```python
from build123d import *

# Parameters (mm, degrees)
SKETCH_1_R      = 3.4
EXTRUDE_1_DEPTH = 120


with BuildPart() as part:
    # 草图1 → 凸台-拉伸1 (new body)
    with BuildSketch(Plane.XY):
        with BuildLine():
            Line((104, 5.1), (105, 5.1))
            Line((105, 5.1), (105, 12.5))
            ThreePointArc((105, 12.5), (104.267766953, 14.267766953), (102.5, 15))
            Line((102.5, 15), (95.1, 15))
            Line((95.1, 15), (95.1, 14))
            Line((95.1, 14), (94.1, 14))
            Line((94.1, 14), (94.1, 12.6))
            Line((94.1, 12.6), (98.25, 12.6))
            Line((98.25, 12.6), (98.25, 10.014213562))
            Line((98.25, 10.014213562), (94.035786438, 5.8))
            Line((94.035786438, 5.8), (85.964213562, 5.8))
            Line((85.964213562, 5.8), (81.75, 10.014213562))
            Line((81.75, 10.014213562), (81.75, 12.6))
            Line((81.75, 12.6), (85.9, 12.6))
            Line((85.9, 12.6), (85.9, 14))
            Line((85.9, 14), (84.9, 14))
            Line((84.9, 14), (84.9, 15))
            Line((84.9, 15), (65.1, 15))
            Line((65.1, 15), (65.1, 14))
            Line((65.1, 14), (64.1, 14))
            Line((64.1, 14), (64.1, 12.6))
            Line((64.1, 12.6), (68.25, 12.6))
            Line((68.25, 12.6), (68.25, 10.014213562))
            Line((68.25, 10.014213562), (64.035786438, 5.8))
            Line((64.035786438, 5.8), (55.964213562, 5.8))
            Line((55.964213562, 5.8), (51.75, 10.014213562))
            Line((51.75, 10.014213562), (51.75, 12.6))
            Line((51.75, 12.6), (55.9, 12.6))
            Line((55.9, 12.6), (55.9, 14))
            Line((55.9, 14), (54.9, 14))
            Line((54.9, 14), (54.9, 15))
            Line((54.9, 15), (35.1, 15))
            Line((35.1, 15), (35.1, 14))
            Line((35.1, 14), (34.1, 14))
            Line((34.1, 14), (34.1, 12.6))
            Line((34.1, 12.6), (38.25, 12.6))
            Line((38.25, 12.6), (38.25, 10.014213562))
            Line((38.25, 10.014213562), (34.035786438, 5.8))
            Line((34.035786438, 5.8), (25.964213562, 5.8))
            Line((25.964213562, 5.8), (21.75, 10.014213562))
            Line((21.75, 10.014213562), (21.75, 12.6))
            Line((21.75, 12.6), (25.9, 12.6))
            Line((25.9, 12.6), (25.9, 14))
            Line((25.9, 14), (24.9, 14))
            Line((24.9, 14), (24.9, 15))
            Line((24.9, 15), (5.1, 15))
            Line((5.1, 15), (5.1, 14))
            Line((5.1, 14), (4.1, 14))
            Line((4.1, 14), (4.1, 12.6))
            Line((4.1, 12.6), (8.25, 12.6))
            Line((8.25, 12.6), (8.25, 10.014213562))
            Line((8.25, 10.014213562), (4.035786438, 5.8))
            Line((4.035786438, 5.8), (-4.035786438, 5.8))
            Line((-4.035786438, 5.8), (-8.25, 10.014213562))
            Line((-8.25, 10.014213562), (-8.25, 12.6))
            Line((-8.25, 12.6), (-4.1, 12.6))
            Line((-4.1, 12.6), (-4.1, 14))
            Line((-4.1, 14), (-5.1, 14))
            Line((-5.1, 14), (-5.1, 15))
            Line((-5.1, 15), (-12.5, 15))
            ThreePointArc((-12.5, 15), (-14.267766953, 14.267766953), (-15, 12.5))
            Line((-15, 12.5), (-15, 5.1))
            Line((-15, 5.1), (-14, 5.1))
            Line((-14, 5.1), (-14, 4.1))
            Line((-14, 4.1), (-12.6, 4.1))
            Line((-12.6, 4.1), (-12.6, 8.25))
            Line((-12.6, 8.25), (-10.014213562, 8.25))
            Line((-10.014213562, 8.25), (-5.8, 4.035786438))
            Line((-5.8, 4.035786438), (-5.8, -4.035786438))
            Line((-5.8, -4.035786438), (-10.014213562, -8.25))
            Line((-10.014213562, -8.25), (-12.6, -8.25))
            Line((-12.6, -8.25), (-12.6, -4.1))
            Line((-12.6, -4.1), (-14, -4.1))
            Line((-14, -4.1), (-14, -5.1))
            Line((-14, -5.1), (-15, -5.1))
            Line((-15, -5.1), (-15, -12.5))
            ThreePointArc((-15, -12.5), (-14.267766953, -14.267766953), (-12.5, -15))
            Line((-12.5, -15), (-5.1, -15))
            Line((-5.1, -15), (-5.1, -14))
            Line((-5.1, -14), (-4.1, -14))
            Line((-4.1, -14), (-4.1, -12.6))
            Line((-4.1, -12.6), (-8.25, -12.6))
            Line((-8.25, -12.6), (-8.25, -10.014213562))
            Line((-8.25, -10.014213562), (-4.035786438, -5.8))
            Line((-4.035786438, -5.8), (4.035786438, -5.8))
            Line((4.035786438, -5.8), (8.25, -10.014213562))
            Line((8.25, -10.014213562), (8.25, -12.6))
            Line((8.25, -12.6), (4.1, -12.6))
            Line((4.1, -12.6), (4.1, -14))
            Line((4.1, -14), (5.1, -14))
            Line((5.1, -14), (5.1, -15))
            Line((5.1, -15), (24.9, -15))
            Line((24.9, -15), (24.9, -14))
            Line((24.9, -14), (25.9, -14))
            Line((25.9, -14), (25.9, -12.6))
            Line((25.9, -12.6), (21.75, -12.6))
            Line((21.75, -12.6), (21.75, -10.014213562))
            Line((21.75, -10.014213562), (25.964213562, -5.8))
            Line((25.964213562, -5.8), (34.035786438, -5.8))
            Line((34.035786438, -5.8), (38.25, -10.014213562))
            Line((38.25, -10.014213562), (38.25, -12.6))
            Line((38.25, -12.6), (34.1, -12.6))
            Line((34.1, -12.6), (34.1, -14))
            Line((34.1, -14), (35.1, -14))
            Line((35.1, -14), (35.1, -15))
            Line((35.1, -15), (54.9, -15))
            Line((54.9, -15), (54.9, -14))
            Line((54.9, -14), (55.9, -14))
            Line((55.9, -14), (55.9, -12.6))
            Line((55.9, -12.6), (51.75, -12.6))
            Line((51.75, -12.6), (51.75, -10.014213562))
            Line((51.75, -10.014213562), (55.964213562, -5.8))
            Line((55.964213562, -5.8), (64.035786438, -5.8))
            Line((64.035786438, -5.8), (68.25, -10.014213562))
            Line((68.25, -10.014213562), (68.25, -12.6))
            Line((68.25, -12.6), (64.1, -12.6))
            Line((64.1, -12.6), (64.1, -14))
            Line((64.1, -14), (65.1, -14))
            Line((65.1, -14), (65.1, -15))
            Line((65.1, -15), (84.9, -15))
            Line((84.9, -15), (84.9, -14))
            Line((84.9, -14), (85.9, -14))
            Line((85.9, -14), (85.9, -12.6))
            Line((85.9, -12.6), (81.75, -12.6))
            Line((81.75, -12.6), (81.75, -10.014213562))
            Line((81.75, -10.014213562), (85.964213562, -5.8))
            Line((85.964213562, -5.8), (94.035786438, -5.8))
            Line((94.035786438, -5.8), (98.25, -10.014213562))
            Line((98.25, -10.014213562), (98.25, -12.6))
            Line((98.25, -12.6), (94.1, -12.6))
            Line((94.1, -12.6), (94.1, -14))
            Line((94.1, -14), (95.1, -14))
            Line((95.1, -14), (95.1, -15))
            Line((95.1, -15), (102.5, -15))
            ThreePointArc((102.5, -15), (104.267766953, -14.267766953), (105, -12.5))
            Line((105, -12.5), (105, -5.1))
            Line((105, -5.1), (104, -5.1))
            Line((104, -5.1), (104, -4.1))
            Line((104, -4.1), (102.6, -4.1))
            Line((102.6, -4.1), (102.6, -8.25))
            Line((102.6, -8.25), (100.014213562, -8.25))
            Line((100.014213562, -8.25), (95.8, -4.035786438))
            Line((95.8, -4.035786438), (95.8, 4.035786438))
            Line((95.8, 4.035786438), (100.014213562, 8.25))
            Line((100.014213562, 8.25), (102.6, 8.25))
            Line((102.6, 8.25), (102.6, 4.1))
            Line((102.6, 4.1), (104, 4.1))
            Line((104, 4.1), (104, 5.1))
        make_face()
        with Locations((90, 0)):
            Circle(SKETCH_1_R, mode=Mode.SUBTRACT)
        with Locations((60, 0)):
            Circle(SKETCH_1_R, mode=Mode.SUBTRACT)
        with Locations((30, 0)):
            Circle(SKETCH_1_R, mode=Mode.SUBTRACT)
        Circle(SKETCH_1_R, mode=Mode.SUBTRACT)
        Polygon((84.2, -4.035786438), (84.2, 4.035786438), (79.25, 8.985786438), (79.25, 12.6), (70.75, 12.6), (70.75, 8.985786438), (65.8, 4.035786438), (65.8, -4.035786438), (70.75, -8.985786438), (70.75, -12.6), (79.25, -12.6), (79.25, -8.985786438), align=None, mode=Mode.SUBTRACT)
        Polygon((54.2, -4.035786438), (54.2, 4.035786438), (49.25, 8.985786438), (49.25, 12.6), (40.75, 12.6), (40.75, 8.985786438), (35.8, 4.035786438), (35.8, -4.035786438), (40.75, -8.985786438), (40.75, -12.6), (49.25, -12.6), (49.25, -8.985786438), align=None, mode=Mode.SUBTRACT)
        Polygon((24.2, -4.035786438), (24.2, 4.035786438), (19.25, 8.985786438), (19.25, 12.6), (10.75, 12.6), (10.75, 8.985786438), (5.8, 4.035786438), (5.8, -4.035786438), (10.75, -8.985786438), (10.75, -12.6), (19.25, -12.6), (19.25, -8.985786438), align=None, mode=Mode.SUBTRACT)
    extrude(amount=EXTRUDE_1_DEPTH)


solid = part.part
```
Model file for the job. Use its own axes, mm. A direction names the side the tool comes from. Coordinates: 2 decimals unless noted, no trailing zeros. Write each loop counter-clockwise with the first axis right and the second up, starting at its lowest first coordinate (ties: lowest second). Pieces come first, ordered by that corner, then holes. Notation, with made-up numbers: (35, 5.25) - (64, 5.25) arc R23 cw to (64, 37.25) - close; hole circle Ø11 at (31.5, 2.25). An arc over 180 degrees is marked (long way). Use a Markdown table: item, result. Add a question column.
Item 1: Band-saw the part on B-B, the plane z = 100.5. Give the number of separate pieces and of enclosed holes in the cut face, and give its area (3 significant figures).
Item 2: Drill centre lines: line 1 along Y through (x, z) = (90, 46); line 2 along Y through (x, z) = (76, 83); line 3 along X through (y, z) = (4.25, 72.5). Where is each one in solid material? Low to high.
Item 3: Drop flat-ended pins along their axis: pin 1 (1.5 mm diameter, centred on x = -13.5, z = 31.5, fed in from -Y); pin 2 (5 mm diameter, centred on x = 2, z = 69, fed in from -Y); pin 3 (10 mm diameter, centred on y = -1.5, z = 77.5, fed in from -X); pin 4 (3 mm diameter, centred on x = 71, y = 7, fed in from -Z). Give the stop position or say it passes through.
Item 4: 3-axis set-ups, long thin cutter, end or side, ignore diameter. For faces 1 (the face through (98.25, -11, 59)), 2 (the face through (0, 5.8, 59)), 3 (the face through (90, -5.8, 59)): which of +Z, -Z, +X, -X, +Y, -Y reach the whole face in a straight line?
Item 5: Two-plate mould, pull along X, no slides. Class faces 4 (the face through (30, 5.8, 59)), 5 (the face through (99, 15, 59)): pulls with the +X half, pulls with the -X half, needs draft (parallel to the pull), parting line crosses it, or undercut.
Item 6: Band-saw the part on A-A, the plane x = 0. Write the cut outline in (y, z).
A:
| question | item | result |
|---|---|---|
| 1 | separate pieces | 1 |
| 1 | enclosed holes | 7 |
| 1 | area | 1,260 mm² |
| 2 | line 1 | y = -5.8 to -3.4, 3.4 to 5.8 |
| 2 | line 2 | y = -15 to -12.6, 12.6 to 15 |
| 2 | line 3 | x = -14 to -12.6, -6.01 to 6.01, 23.99 to 36.01, 53.99 to 66.01, 83.99 to 96.01, 102.6 to 104 |
| 3 | pin 1 | stops at y = -14.99 |
| 3 | pin 2 | stops at y = -14 |
| 3 | pin 3 | stops at x = -15 |
| 3 | pin 4 | passes through |
| 4 | face 1 | +Z, -Z |
| 4 | face 2 | +Z, -Z, +Y |
| 4 | face 3 | +Z, -Z, -Y |
| 5 | face 4 | undercut |
| 5 | face 5 | needs draft |
| 6 | outline | (-5.8, 0) - (-3.4, 0) - (-3.4, 120) - (-5.8, 120) - close; (3.4, 0) - (5.8, 0) - (5.8, 120) - (3.4, 120) - close |
